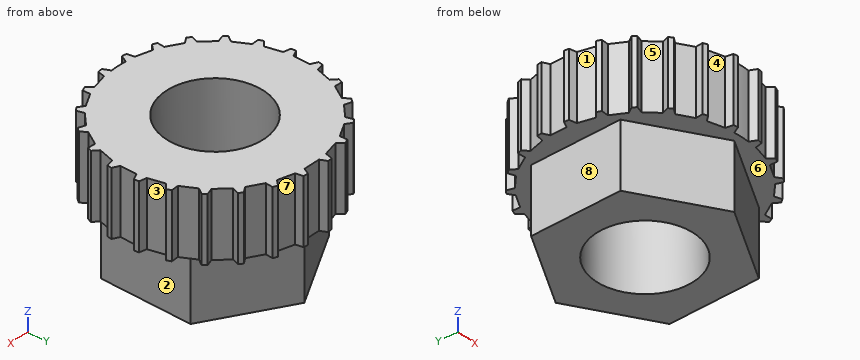
Autodesk Inventor part; units mm, degrees
ref_plane "YZ Plane" through (0, 0, 0) normal (1, 0, 0) x (0, 1, 0)
ref_plane "XZ Plane" through (0, 0, 0) normal (0, 1, 0) x (-1, 0, 0)
ref_plane "XY Plane" through (0, 0, 0) normal (0, 0, 1) x (1, 0, 0)
sketch "Sketch1" plane through (0, 0, 0) normal (0, 0, 1) x (1, 0, 0)
  circle A0 centre (0, 0) radius 17.25
  circle A1 centre (0, 0) radius 16.1
  circle A2 centre (0, 0) radius 15
  line L0 (-1.25, -15.0046) -> (1.25, -15.0046)
  line L1 (-1.75, -16.0046) -> (1.75, -16.0046)
  line L2 (1.75, -16.0046) -> (1.25, -15.0046)
  line L3 (-1.75, -16.0046) -> (-1.25, -15.0046)
  line L4 (-1.25, -15.0046) -> (-1.2227, -14.9501)
  line L5 (1.25, -15.0046) -> (1.2227, -14.9501)
  line L6 (2.6761, -14.8169) -> (5.0909, -14.1698)
  line L7 (2.4519, -15.9122) -> (2.6761, -14.8169)
  line L8 (2.6761, -14.8169) -> (2.6883, -14.7571)
  line L9 (5.8327, -15.0063) -> (5.0909, -14.1698)
  line L10 (5.0909, -14.1698) -> (5.0504, -14.1242)
  line L11 (6.4198, -13.6194) -> (8.5848, -12.3694)
  line L12 (6.4868, -14.7354) -> (6.4198, -13.6194)
  line L13 (6.4198, -13.6194) -> (6.4161, -13.5585)
  line L14 (9.5178, -12.9854) -> (8.5848, -12.3694)
  line L15 (8.5848, -12.3694) -> (8.534, -12.3358)
  line L16 (9.726, -11.4937) -> (11.4937, -9.726)
  line L17 (10.0795, -12.5544) -> (9.726, -11.4937)
  line L18 (9.726, -11.4937) -> (9.7067, -11.4359)
  line L19 (12.5544, -10.0795) -> (11.4937, -9.726)
  line L20 (11.4937, -9.726) -> (11.4359, -9.7067)
  line L21 (12.3694, -8.5848) -> (13.6194, -6.4198)
  line L22 (12.9854, -9.5178) -> (12.3694, -8.5848)
  line L23 (12.3694, -8.5848) -> (12.3358, -8.534)
  line L24 (14.7354, -6.4868) -> (13.6194, -6.4198)
  line L25 (13.6194, -6.4198) -> (13.5585, -6.4161)
  line L26 (14.1698, -5.0909) -> (14.8169, -2.6761)
  line L27 (15.0063, -5.8327) -> (14.1698, -5.0909)
  line L28 (14.1698, -5.0909) -> (14.1242, -5.0504)
  line L29 (15.9122, -2.4519) -> (14.8169, -2.6761)
  line L30 (14.8169, -2.6761) -> (14.7571, -2.6883)
  line L31 (15.0046, -1.25) -> (15.0046, 1.25)
  line L32 (16.0046, -1.75) -> (15.0046, -1.25)
  line L33 (15.0046, -1.25) -> (14.9501, -1.2227)
  line L34 (16.0046, 1.75) -> (15.0046, 1.25)
  line L35 (15.0046, 1.25) -> (14.9501, 1.2227)
  line L36 (14.8169, 2.6761) -> (14.1698, 5.0909)
  line L37 (15.9122, 2.4519) -> (14.8169, 2.6761)
  line L38 (14.8169, 2.6761) -> (14.7571, 2.6883)
  line L39 (15.0063, 5.8327) -> (14.1698, 5.0909)
  line L40 (14.1698, 5.0909) -> (14.1242, 5.0504)
  line L41 (13.6194, 6.4198) -> (12.3694, 8.5848)
  line L42 (14.7354, 6.4868) -> (13.6194, 6.4198)
  line L43 (13.6194, 6.4198) -> (13.5585, 6.4161)
  line L44 (12.9854, 9.5178) -> (12.3694, 8.5848)
  line L45 (12.3694, 8.5848) -> (12.3358, 8.534)
  line L46 (11.4937, 9.726) -> (9.726, 11.4937)
  line L47 (12.5544, 10.0795) -> (11.4937, 9.726)
  line L48 (11.4937, 9.726) -> (11.4359, 9.7067)
  line L49 (10.0795, 12.5544) -> (9.726, 11.4937)
  line L50 (9.726, 11.4937) -> (9.7067, 11.4359)
  line L51 (8.5848, 12.3694) -> (6.4198, 13.6194)
  line L52 (9.5178, 12.9854) -> (8.5848, 12.3694)
  line L53 (8.5848, 12.3694) -> (8.534, 12.3358)
  line L54 (6.4868, 14.7354) -> (6.4198, 13.6194)
  line L55 (6.4198, 13.6194) -> (6.4161, 13.5585)
  line L56 (5.0909, 14.1698) -> (2.6761, 14.8169)
  line L57 (5.8327, 15.0063) -> (5.0909, 14.1698)
  line L58 (5.0909, 14.1698) -> (5.0504, 14.1242)
  line L59 (2.4519, 15.9122) -> (2.6761, 14.8169)
  line L60 (2.6761, 14.8169) -> (2.6883, 14.7571)
  line L61 (1.25, 15.0046) -> (-1.25, 15.0046)
  line L62 (1.75, 16.0046) -> (1.25, 15.0046)
  line L63 (1.25, 15.0046) -> (1.2227, 14.9501)
  line L64 (-1.75, 16.0046) -> (-1.25, 15.0046)
  line L65 (-1.25, 15.0046) -> (-1.2227, 14.9501)
  line L66 (-2.6761, 14.8169) -> (-5.0909, 14.1698)
  line L67 (-2.4519, 15.9122) -> (-2.6761, 14.8169)
  line L68 (-2.6761, 14.8169) -> (-2.6883, 14.7571)
  line L69 (-5.8327, 15.0063) -> (-5.0909, 14.1698)
  line L70 (-5.0909, 14.1698) -> (-5.0504, 14.1242)
  line L71 (-6.4198, 13.6194) -> (-8.5848, 12.3694)
  line L72 (-6.4868, 14.7354) -> (-6.4198, 13.6194)
  line L73 (-6.4198, 13.6194) -> (-6.4161, 13.5585)
  line L74 (-9.5178, 12.9854) -> (-8.5848, 12.3694)
  line L75 (-8.5848, 12.3694) -> (-8.534, 12.3358)
  line L76 (-9.726, 11.4937) -> (-11.4937, 9.726)
  line L77 (-10.0795, 12.5544) -> (-9.726, 11.4937)
  line L78 (-9.726, 11.4937) -> (-9.7067, 11.4359)
  line L79 (-12.5544, 10.0795) -> (-11.4937, 9.726)
  line L80 (-11.4937, 9.726) -> (-11.4359, 9.7067)
  line L81 (-12.3694, 8.5848) -> (-13.6194, 6.4198)
  line L82 (-12.9854, 9.5178) -> (-12.3694, 8.5848)
  line L83 (-12.3694, 8.5848) -> (-12.3358, 8.534)
  line L84 (-14.7354, 6.4868) -> (-13.6194, 6.4198)
  line L85 (-13.6194, 6.4198) -> (-13.5585, 6.4161)
  line L86 (-14.1698, 5.0909) -> (-14.8169, 2.6761)
  line L87 (-15.0063, 5.8327) -> (-14.1698, 5.0909)
  line L88 (-14.1698, 5.0909) -> (-14.1242, 5.0504)
  line L89 (-15.9122, 2.4519) -> (-14.8169, 2.6761)
  line L90 (-14.8169, 2.6761) -> (-14.7571, 2.6883)
  line L91 (-15.0046, 1.25) -> (-15.0046, -1.25)
  line L92 (-16.0046, 1.75) -> (-15.0046, 1.25)
  line L93 (-15.0046, 1.25) -> (-14.9501, 1.2227)
  line L94 (-16.0046, -1.75) -> (-15.0046, -1.25)
  line L95 (-15.0046, -1.25) -> (-14.9501, -1.2227)
  line L96 (-14.8169, -2.6761) -> (-14.1698, -5.0909)
  line L97 (-15.9122, -2.4519) -> (-14.8169, -2.6761)
  line L98 (-14.8169, -2.6761) -> (-14.7571, -2.6883)
  line L99 (-15.0063, -5.8327) -> (-14.1698, -5.0909)
  line L100 (-14.1698, -5.0909) -> (-14.1242, -5.0504)
  line L101 (-13.6194, -6.4198) -> (-12.3694, -8.5848)
  line L102 (-14.7354, -6.4868) -> (-13.6194, -6.4198)
  line L103 (-13.6194, -6.4198) -> (-13.5585, -6.4161)
  line L104 (-12.9854, -9.5178) -> (-12.3694, -8.5848)
  line L105 (-12.3694, -8.5848) -> (-12.3358, -8.534)
  line L106 (-11.4937, -9.726) -> (-9.726, -11.4937)
  line L107 (-12.5544, -10.0795) -> (-11.4937, -9.726)
  line L108 (-11.4937, -9.726) -> (-11.4359, -9.7067)
  line L109 (-10.0795, -12.5544) -> (-9.726, -11.4937)
  line L110 (-9.726, -11.4937) -> (-9.7067, -11.4359)
  line L111 (-8.5848, -12.3694) -> (-6.4198, -13.6194)
  line L112 (-9.5178, -12.9854) -> (-8.5848, -12.3694)
  line L113 (-8.5848, -12.3694) -> (-8.534, -12.3358)
  line L114 (-6.4868, -14.7354) -> (-6.4198, -13.6194)
  line L115 (-6.4198, -13.6194) -> (-6.4161, -13.5585)
  line L116 (-5.0909, -14.1698) -> (-2.6761, -14.8169)
  line L117 (-5.8327, -15.0063) -> (-5.0909, -14.1698)
  line L118 (-5.0909, -14.1698) -> (-5.0504, -14.1242)
  line L119 (-2.4519, -15.9122) -> (-2.6761, -14.8169)
  line L120 (-2.6761, -14.8169) -> (-2.6883, -14.7571)
  point P0 (0, -16.0046)
  point P1 (0, -15.0046)
  point P2 (1.75, -16.0046)
  point P3 (3.8835, -14.4933)
  point P4 (7.5023, -12.9944)
  point P5 (10.6099, -10.6099)
  point P6 (12.9944, -7.5023)
  point P7 (14.4933, -3.8835)
  point P8 (15.0046, 0)
  point P9 (14.4933, 3.8835)
  point P10 (12.9944, 7.5023)
  point P11 (10.6099, 10.6099)
  point P12 (7.5023, 12.9944)
  point P13 (3.8835, 14.4933)
  point P14 (0, 15.0046)
  point P15 (-3.8835, 14.4933)
  point P16 (-7.5023, 12.9944)
  point P17 (-10.6099, 10.6099)
  point P18 (-12.9944, 7.5023)
  point P19 (-14.4933, 3.8835)
  point P20 (-15.0046, 0)
  point P21 (-14.4933, -3.8835)
  point P22 (-12.9944, -7.5023)
  point P23 (-10.6099, -10.6099)
  point P24 (-7.5023, -12.9944)
  point P25 (-3.8835, -14.4933)
  dimension "d1" = 32.2
  dimension "d0" = 34.5
  dimension "d2" = 30
  dimension "d3" = 2.5
  dimension "d4" = 3.5
  dimension "d5" = 1
  dimension "d20" = 360
extrude "Extrusion1" add sketch "Sketch1" along normal blind 10 contours L34 L35 A2 L38 L37 A1 | A1 L29 L30 A2 L33 L32 | L31 L33 A2 L35 | L39 L40 A2 L43 L42 A1 | L38 A2 L40 L36 | A2 | A1 L24 L25 A2 L28 L27 | L26 L28 A2 L30 | L44 L45 A2 L48 L47 A1 | L43 A2 L45 L41 | A1 L19 L20 A2 L23 L22 | L21 L23 A2 L25 | L49 L50 A2 L53 L52 A1 | L48 A2 L50 L46 | A1 L14 L15 A2 L18 L17 | L16 L18 A2 L20 | L54 L55 A2 L58 L57 A1 | L53 A2 L55 L51 | A1 L9 L10 A2 L13 L12 | L11 L13 A2 L15 | L59 L60 A2 L63 L62 A1 | L58 A2 L60 L56 | A1 L2 L5 A2 L8 L7 | L6 L8 A2 L10 | L64 L65 A2 L68 L67 A1 | L63 A2 L65 L61 | A1 L119 L120 A2 L4 L3 | L69 L70 A2 L73 L72 A1 | L68 A2 L70 L66 | A1 L114 L115 A2 L118 L117 | L116 L118 A2 L120 | L74 L75 A2 L78 L77 A1 | L73 A2 L75 L71 | A1 L109 L110 A2 L113 L112 | L111 L113 A2 L115 | L79 L80 A2 L83 L82 A1 | L78 A2 L80 L76 | A1 L104 L105 A2 L108 L107 | L106 L108 A2 L110 | L84 L85 A2 L88 L87 A1 | L83 A2 L85 L81 | A1 L99 L100 A2 L103 L102 | L101 L103 A2 L105 | L89 L90 A2 L93 L92 A1 | L88 A2 L90 L86 | A1 L94 L95 A2 L98 L97 | L96 L98 A2 L100 | L93 A2 L95 L91
sketch "Sketch2" plane through (0, 0, 0) normal (0, 0, -1) x (-1, 0, 0)
  line L0 (12, 6.9282) -> (12, -6.9282)
  line L1 (12, -6.9282) -> (0, -13.8564)
  line L2 (0, -13.8564) -> (-12, -6.9282)
  line L3 (-12, -6.9282) -> (-12, 6.9282)
  line L4 (-12, 6.9282) -> (0, 13.8564)
  line L5 (0, 13.8564) -> (12, 6.9282)
  point P0 (0, 0)
  point P1 (0, 0)
  dimension "d12" = 24
extrude "Extrusion2" add sketch "Sketch2" along normal blind 10
sketch "Sketch3" plane through (0, 0, -10) normal (0, 0, -1) x (-1, 0, 0)
  circle A0 centre (0, 0) radius 7.5
  dimension "d15" = 15
extrude "Extrusion3" cut sketch "Sketch3" against normal up to surface (20 mm away)
properties part number "Nastavek Millard freewheel tool"
Could you check a few things on this model? Use its own coordinates, in mm. Face numbers are marked on the shaded views. A direction names the side the tool comes from. Give positions to 0.01 mm unless a question says otherwise; leave off trailing zeros. Loops run counter-clockwise (first coordinate to the right, second up) from the corner with the lowest first, then second, coordinate; pieces in that order, holes last. Notation, with made-up numbers: (29, -38.5) -> (40, -38.5) arc R34 ccw to (40, -8.5) -> close; hole circle Ø5 at (-39.75, 14). An arc over 180 degrees is marked (long way). Return JSON: item names as keys, results as strings.
Item 1: If we section it at C-C on x = -7: List the corners of the cut face in (y, z) for me.
Geometry results:
{"outline": "(-13.28, 0) -> (-9.81, 0) -> (-9.81, -10) -> (-2.69, -10) -> (-2.69, 10) -> (-13.28, 10) -> close; (2.69, -10) -> (9.81, -10) -> (9.81, 0) -> (13.28, 0) -> (13.28, 10) -> (2.69, 10) -> close"}
Item 2: I'm going to push flat-ended pins straight in: pin 1 (0.8 mm diameter, centred on y = 0, z = 2.5, fed in from +X); pin 2 (4 mm diameter, centred on x = -7, z = -6, fed in from +Y); pin 3 (6 mm diameter, centred on x = -6.5, z = 4.5, fed in from -Y); pin 4 (12 mm diameter, centred on x = 0, y = 0, fed in from +Z). Where does each tip first touch, or does it pass through?
Geometry results:
{"pin 1": "stops at x = 15", "pin 2": "stops at y = 10.97", "pin 3": "stops at y = -15.01", "pin 4": "passes through"}
Item 3: I need wall thicknesses on L1, parallel to Y at x = 0, z = -4; L2, parallel to Y at x = 0, z = 3.75; L3, parallel to X at y = -12.5, z = 9.25. Which ranges of each line are inside material? Lowest first, please. Write a range as from..to.
Geometry results:
{"L1": "y = -13.86..-7.5, 7.5..13.86", "L2": "y = -15..-7.5, 7.5..15", "L3": "x = -10.06..-8.78, -8.36..8.36, 8.78..10.06"}
Item 4: If we section it at A-A on z = -2.25: List the corners of the cut face in (x, y) for me.
Geometry results:
{"outline": "(-12, -6.93) -> (0, -13.86) -> (12, -6.93) -> (12, 6.93) -> (0, 13.86) -> (-12, 6.93) -> close; hole circle Ø15 at (0, 0)"}
Item 5: Which directions (+Z, -Z, +X, -X, +Y, -Y) give clear straight access to the entire face, cutting with the end or side of a thin tool? Please do the marked faces 1, 2, 3, 4 and 5.
Geometry results:
{"face 1": "+Z, -Z, -X", "face 2": "-Z, +X, +Y, -Y", "face 3": "+Z, -Z, +X", "face 4": "+Z, -Z, -Y", "face 5": "+Z, -Z"}
Item 6: If we section it at B-B on y = 0: List the corners of the cut face in (x, z) for me, plus the area to 3 significant figures.
Geometry results:
{"outline": "(-15, 0) -> (-12, 0) -> (-12, -10) -> (-7.5, -10) -> (-7.5, 10) -> (-15, 10) -> close; (7.5, -10) -> (12, -10) -> (12, 0) -> (15, 0) -> (15, 10) -> (7.5, 10) -> close", "area": "240 mm²"}
Item 7: We'd pull the mould along X, two halves only. Please class the marked faces 6, 7 and 8: +X half, -X half, draft (parallel to the pull), parting line (faces both ways), or undercut.
Geometry results:
{"face 6": "draft", "face 7": "undercut", "face 8": "-X half"}
